```python
from build123d import *

# Parameters (mm, degrees)
BLANKSKE_W         = 41.5
BLANKSKE_H         = 2.6
BLANK_DEPTH        = 5
TOOTHCUTSIM_DEPTH  = 42.880902569
TEETHCUTS_COUNT    = 23
TEETHCUTS_PITCH    = 1.88495559
CUT_EXTRUDE1_DEPTH = 0.2
CUT_EXTRUDE2_DEPTH = 0.2


with BuildPart() as part:
    # BlankSke → Blank (new body)
    with BuildSketch(Plane.XY):
        with Locations((20.75, 1.3)):
            Rectangle(BLANKSKE_W, BLANKSKE_H)
    extrude(amount=-BLANK_DEPTH)

    # TooCutSkeSim → ToothCutSim (cut, through all)
    with BuildSketch(Plane.XY):
        Polygon((0.267261222, 1.25), (-0.267261222, 1.25), (-0.767865882, 2.6254), (0.767865882, 2.6254), align=None)
    toothcutsim = extrude(amount=-TOOTHCUTSIM_DEPTH, mode=Mode.SUBTRACT)

    # TeethCuts: ToothCutSim ×23
    with Locations(*[(i * TEETHCUTS_PITCH, 0, 0) for i in range(1, TEETHCUTS_COUNT)]):
        add(toothcutsim, mode=Mode.SUBTRACT)

    # Sketch1 → Cut-Extrude1 (cut)
    with BuildSketch(Plane.XY):
        Polygon((41.5, 1.25), (41.201761758, 1.25), (40.710401942, 2.6), (40.342688428, 2.6), (39.851328612, 1.25), (39.316806168, 1.25), (38.825446352, 2.6), (38.457732838, 2.6), (37.966373022, 1.25), (37.431850578, 1.25), (36.940490762, 2.6), (36.572777248, 2.6), (36.081417432, 1.25), (35.546894988, 1.25), (35.055535172, 2.6), (34.687821658, 2.6), (34.196461842, 1.25), (33.661939398, 1.25), (33.170579582, 2.6), (32.802866068, 2.6), (32.311506252, 1.25), (31.776983808, 1.25), (31.285623992, 2.6), (30.917910478, 2.6), (30.426550662, 1.25), (29.892028218, 1.25), (29.400668402, 2.6), (29.032954888, 2.6), (28.541595072, 1.25), (28.007072628, 1.25), (27.515712812, 2.6), (27.147999298, 2.6), (26.656639482, 1.25), (26.122117038, 1.25), (25.630757222, 2.6), (25.263043708, 2.6), (24.771683892, 1.25), (24.237161448, 1.25), (23.745801632, 2.6), (23.378088118, 2.6), (22.886728302, 1.25), (22.352205858, 1.25), (21.860846042, 2.6), (21.493132528, 2.6), (21.001772712, 1.25), (20.467250268, 1.25), (19.975890452, 2.6), (19.608176938, 2.6), (19.116817122, 1.25), (18.582294678, 1.25), (18.090934862, 2.6), (17.723221348, 2.6), (17.231861532, 1.25), (16.697339088, 1.25), (16.205979272, 2.6), (15.838265758, 2.6), (15.346905942, 1.25), (14.812383498, 1.25), (14.321023682, 2.6), (13.953310168, 2.6), (13.461950352, 1.25), (12.927427908, 1.25), (12.436068092, 2.6), (12.068354578, 2.6), (11.576994762, 1.25), (11.042472318, 1.25), (10.551112502, 2.6), (10.183398988, 2.6), (9.692039172, 1.25), (9.157516728, 1.25), (8.666156912, 2.6), (8.298443398, 2.6), (7.807083582, 1.25), (7.272561138, 1.25), (6.781201322, 2.6), (6.413487808, 2.6), (5.922127992, 1.25), (5.387605548, 1.25), (4.896245732, 2.6), (4.528532218, 2.6), (4.037172402, 1.25), (3.502649958, 1.25), (3.011290142, 2.6), (2.643576628, 2.6), (2.152216812, 1.25), (1.617694368, 1.25), (1.126334552, 2.6), (0.758621038, 2.6), (0.267261222, 1.25), (0, 1.25), (0, 0), (41.5, 0), align=None)
    extrude(amount=-CUT_EXTRUDE1_DEPTH, mode=Mode.SUBTRACT)

    # Sketch2 → Cut-Extrude2 (cut)
    with BuildSketch(Plane(origin=(0, 0, -5), x_dir=(-1, 0, 0), z_dir=(0, 0, -1))):
        Polygon((-40.710401942, 2.6), (-41.201761758, 1.25), (-41.5, 1.25), (-41.5, 0), (0, 0), (0, 1.25), (-0.267261222, 1.25), (-0.758621038, 2.6), (-1.126334552, 2.6), (-1.617694368, 1.25), (-2.152216812, 1.25), (-2.643576628, 2.6), (-3.011290142, 2.6), (-3.502649958, 1.25), (-4.037172402, 1.25), (-4.528532218, 2.6), (-4.896245732, 2.6), (-5.387605548, 1.25), (-5.922127992, 1.25), (-6.413487808, 2.6), (-6.781201322, 2.6), (-7.272561138, 1.25), (-7.807083582, 1.25), (-8.298443398, 2.6), (-8.666156912, 2.6), (-9.157516728, 1.25), (-9.692039172, 1.25), (-10.183398988, 2.6), (-10.551112502, 2.6), (-11.042472318, 1.25), (-11.576994762, 1.25), (-12.068354578, 2.6), (-12.436068092, 2.6), (-12.927427908, 1.25), (-13.461950352, 1.25), (-13.953310168, 2.6), (-14.321023682, 2.6), (-14.812383498, 1.25), (-15.346905942, 1.25), (-15.838265758, 2.6), (-16.205979272, 2.6), (-16.697339088, 1.25), (-17.231861532, 1.25), (-17.723221348, 2.6), (-18.090934862, 2.6), (-18.582294678, 1.25), (-19.116817122, 1.25), (-19.608176938, 2.6), (-19.975890452, 2.6), (-20.467250268, 1.25), (-21.001772712, 1.25), (-21.493132528, 2.6), (-21.860846042, 2.6), (-22.352205858, 1.25), (-22.886728302, 1.25), (-23.378088118, 2.6), (-23.745801632, 2.6), (-24.237161448, 1.25), (-24.771683892, 1.25), (-25.263043708, 2.6), (-25.630757222, 2.6), (-26.122117038, 1.25), (-26.656639482, 1.25), (-27.147999298, 2.6), (-27.515712812, 2.6), (-28.007072628, 1.25), (-28.541595072, 1.25), (-29.032954888, 2.6), (-29.400668402, 2.6), (-29.892028218, 1.25), (-30.426550662, 1.25), (-30.917910478, 2.6), (-31.285623992, 2.6), (-31.776983808, 1.25), (-32.311506252, 1.25), (-32.802866068, 2.6), (-33.170579582, 2.6), (-33.661939398, 1.25), (-34.196461842, 1.25), (-34.687821658, 2.6), (-35.055535172, 2.6), (-35.546894988, 1.25), (-36.081417432, 1.25), (-36.572777248, 2.6), (-36.940490762, 2.6), (-37.431850578, 1.25), (-37.966373022, 1.25), (-38.457732838, 2.6), (-38.825446352, 2.6), (-39.316806168, 1.25), (-39.851328612, 1.25), (-40.342688428, 2.6), align=None)
    extrude(amount=-CUT_EXTRUDE2_DEPTH, mode=Mode.SUBTRACT)


solid = part.part
```
Here's how the part is built. I have some questions about the finished solid (model axes, mm). A direction names the side the tool comes from. Give positions to 0.01 mm unless a question says otherwise; leave off trailing zeros. Use one line per item in the form item = value. Start each with the question number.
1) Thinking about a two-plate mould opening in X: for faces 1 (the face through (18.34, 1.92, -2.47)), 2 (the face through (21, 1, -4.8)), 3 (the face through (23.136, 1.934, -2.468)), 4 (the face through (0, 1, -2)), which applies, +X half, -X half, draft (parallel to the pull), parting line (faces both ways), or undercut?
2) Imagine slicing it at A-A (y = 1.8). Count the separate pieces of the cut face and the enclosed holes in it, then the cut area to 3 significant figures.
3) Which directions (+Z, -Z, +X, -X, +Y, -Y) give clear straight access to the entire face, cutting with the end or side of a thin tool? Please do faces 5 (the face through (20, 1, -0.2)), 6 (the face through (15.596, 1.934, -2.468)).
4) Please list where this line runs through material, in increasing order: line 1 along Y through (x, z) = (39.5, -3).
Check values:
q1.face_1 = undercut
q1.face_2 = draft
q1.face_3 = undercut
q1.face_4 = -X half
q2.separate_pieces = 22
q2.enclosed_holes = 0
q2.area = 96.1 mm^2
q3.face_5 = +Z, +X, -X, +Y, -Y
q3.face_6 = +Z, -Z, +Y
q4.line_1 = 0 to 1.25
